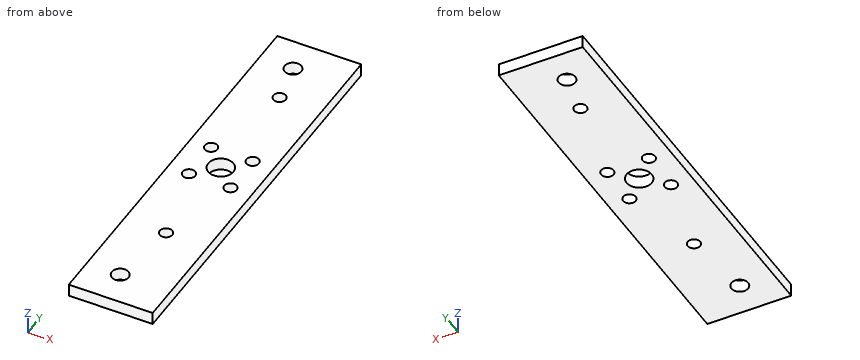
```python
from build123d import *

# Parameters (mm, degrees)
SKETCH_1_W           = 170.943732818
SKETCH_1_H           = 105.520822726
EXTRUDE_1_DEPTH      = 3
SKETCH_3_OUTSIDE_W   = 213.126
SKETCH_3_OUTSIDE_H   = 147.702
SKETCH_3_OUTSIDE_W_2 = 20
SKETCH_3_OUTSIDE_H_2 = 88.50002898
CUT_EXTRUDE_1_DEPTH  = 101.489307663
SKETCH_2_R           = 1.5
SKETCH_2_R_2         = 3
CUT_EXTRUDE_2_DEPTH  = 58.243779886
SKETCH_4_R           = 1.5
CUT_EXTRUDE_3_DEPTH  = 58.243779886
SKETCH_9_W           = 20
SKETCH_9_H           = 3
EXTRUDE_3_DEPTH      = 5
SKETCH_10_W          = 20
SKETCH_10_H          = 3
EXTRUDE_4_DEPTH      = 5
SKETCH_11_R          = 2
CUT_EXTRUDE_4_DEPTH  = 5


with BuildPart() as part:
    # 草图1 → 凸台-拉伸1 (new body)
    with BuildSketch(Plane.XY):
        Rectangle(SKETCH_1_W, SKETCH_1_H)
    extrude(amount=EXTRUDE_1_DEPTH)

    # 草图3 outside → 切除-拉伸1 (cut, through all)
    with BuildSketch(Plane.XY.offset(3)):
        Rectangle(SKETCH_3_OUTSIDE_W, SKETCH_3_OUTSIDE_H)
        with Locations((-12.004302498, 13.711132511)):
            Rectangle(SKETCH_3_OUTSIDE_W_2, SKETCH_3_OUTSIDE_H_2, mode=Mode.SUBTRACT)
    extrude(amount=-CUT_EXTRUDE_1_DEPTH, mode=Mode.SUBTRACT)

    # 草图2 → 切除-拉伸2 (cut, through all)
    with BuildSketch(Plane(origin=(0, 0, 0), x_dir=(-1, 0, 0), z_dir=(0, 0, -1))):
        with Locations((7.05455503, 18.660879979)):
            Circle(SKETCH_2_R)
        with Locations((16.954049967, 18.660879979)):
            Circle(SKETCH_2_R)
        with Locations((16.954049967, 8.761385043)):
            Circle(SKETCH_2_R)
        with Locations((7.05455503, 8.761385043)):
            Circle(SKETCH_2_R)
        with Locations((12.004302498, 13.711132511)):
            Circle(SKETCH_2_R_2)
    extrude(amount=-CUT_EXTRUDE_2_DEPTH, mode=Mode.SUBTRACT)

    # 草图4 → 切除-拉伸3 (cut, through all)
    with BuildSketch(Plane(origin=(0, 0, 0), x_dir=(-1, 0, 0), z_dir=(0, 0, -1))):
        with Locations((12.004302498, 40.007436866)):
            Circle(SKETCH_4_R)
        with Locations((12.004302498, -10.785171844)):
            Circle(SKETCH_4_R)
    extrude(amount=-CUT_EXTRUDE_3_DEPTH, mode=Mode.SUBTRACT)

    # 草图9 → 凸台-拉伸3 (add)
    with BuildSketch(Plane(origin=(0, 52.760411363, 0), x_dir=(1, 0, 0), z_dir=(0, 1, 0))):
        with Locations((-12.004302498, -1.5)):
            Rectangle(SKETCH_9_W, SKETCH_9_H)
    extrude(amount=EXTRUDE_3_DEPTH)

    # 草图10 → 凸台-拉伸4 (add)
    with BuildSketch(Plane.XZ.offset(30.538881979)):
        with Locations((-12.004302498, 1.5)):
            Rectangle(SKETCH_10_W, SKETCH_10_H)
    extrude(amount=EXTRUDE_4_DEPTH)

    # 草图11 → 切除-拉伸4 (cut)
    with BuildSketch(Plane.XY.offset(3)):
        with Locations((-14.004302498, 49.760411363)):
            Circle(SKETCH_11_R)
        with Locations((-14.004302498, -27.538881979)):
            Circle(SKETCH_11_R)
    extrude(amount=-CUT_EXTRUDE_4_DEPTH, mode=Mode.SUBTRACT)


solid = part.part
```
The listing builds one solid part. Answer for the finished solid, in the listing's coordinates (mm). Give positions to 0.01 mm unless a question says otherwise; leave off trailing zeros. Order: outer loops, then holes, each group sorted by start corner. A loop starts at its lowest first (then second) coordinate and runs counter-clockwise, first axis right, second up. Notation, with made-up numbers: (3, -13) - (42, -13) arc R23 cw to (42, 19) - close; hole circle Ø11 at (-25, 0.5). An arc over 180 degrees is marked (long way). Answer in a Markdown table with one row per item. Add a question column.
Q1. The part is cut by section A-A (z = 1.4). Give the number of separate pieces and of enclosed holes in the cut face, then the cut area to 3 significant figures.
Q2. Find the intervals of material crossed by line 1 along Y through (x, z) = (-7.25, 1.05); line 2 along X through (y, z) = (9, 2.5); line 3 along X through (y, z) = (14, 2.65), in increasing order. Write a range as [from, to].
Q3. The part is cut by section B-B (x = -6.5). Determine the outline of the cut face in (y, z).
Q4. Given P1, Ø2.5, axis at x = -7.05, y = 18.66, coming from the -Z side, flat-ended and moving along its own axis, determine where the tip first touches the part or whether it passes through.
Determined:
| question | item | result |
|---|---|---|
| 1 | separate pieces | 1 |
| 1 | enclosed holes | 9 |
| 1 | area | 1,770 mm² |
| 2 | line 1 | y = [-35.54, 7.27], [10.25, 17.17], [20.15, 57.76] |
| 2 | line 2 | x = [-22, -18.43], [-15.47, -8.54], [-5.57, -2] |
| 2 | line 3 | x = [-22, -14.99], [-9.02, -2] |
| 3 | outline | (-35.54, 0) - (7.37, 0) - (7.37, 3) - (-35.54, 3) - close; (10.16, 0) - (17.27, 0) - (17.27, 3) - (10.16, 3) - close; (20.05, 0) - (57.76, 0) - (57.76, 3) - (20.05, 3) - close |
| 4 | P1 | passes through |
